For this review, take the finished solid that the model builds, in its own axes (mm). Round coordinates to 2 decimals unless told otherwise and drop trailing zeros. Order: outer loops, then holes, each group sorted by start corner. A loop starts at its lowest first (then second) coordinate and runs counter-clockwise, first axis right, second up. Notation, with made-up numbers: (61, -10.5) - (112, -10.5) arc R14 cw to (112, 5.5) - close; hole circle Ø7 at (-23, 53.5). An arc over 180 degrees is marked (long way). One line per question, with ' | ' between items.
```python
from build123d import *

# Parameters (mm, degrees)
SKETCH1_R           = 6
BOSS_EXTRUDE1_DEPTH = 6


with BuildPart() as part:
    # Sketch1 → Boss-Extrude1 (new body)
    with BuildSketch(Plane(origin=(0, 0, 0), x_dir=(1, 0, 0), z_dir=(0, 1, 0))):
        with BuildLine():
            Line((8.845195956, 114.659332409), (0, 0))
            Line((0, 0), (49.851883656, -3.845737372))
            Line((49.851883656, -3.845737372), (49.851883656, 10.382317327))
            Line((49.851883656, 10.382317327), (18.624081043, 115.696191659))
            ThreePointArc((18.624081043, 115.696191659), (13.303187452, 119.246887337), (8.845195956, 114.659332409))
        make_face()
        with Locations((16.515553245, 88.289115087)):
            Circle(SKETCH1_R, mode=Mode.SUBTRACT)
    extrude(amount=BOSS_EXTRUDE1_DEPTH)


solid = part.part
```
(1) Insertion check: pin 1 (3 mm diameter, centred on y = 4.5, z = -40.5, fed in from +X). The pin has a flat end and moves straight along its axis. Give the tip position at first contact, or say it passes through.
Output values:
pin 1: x = 41.37
(2) For probe 1 along X at (y, z) = (0.9, -89); probe 2 along X at (y, z) = (0.8, -85.5); probe 3 along Z at (x, y) = (12.5, 0.95), list the stretches that pass through material, from the lowest coordinate up. Write a range as [from, to].
Output values:
probe 1: [6.87, 10.56], [22.47, 26.54] | probe 2: [6.6, 11.2], [21.83, 27.58] | probe 3: [-119.09, -92.75], [-83.83, 0.96]
(3) We need section A-A on x = 21. State the section outline as (y, z) points.
Output values:
outline: (0, -107.68) - (6, -107.68) - (6, -92.28) - (0, -92.28) - close; (0, -84.3) - (6, -84.3) - (6, 1.62) - (0, 1.62) - close
(4) We need section C-C on z = -15. State the section outline as (x, y) points, plus the area to 3 significant figures.
Output values:
outline: (1.16, 0) - (48.48, 0) - (48.48, 6) - (1.16, 6) - close | area: 284 mm^2
(5) Mouldability with a two-part tool opening along X and no side actions: class faces 1 (the flat face through (19, 6, -45)), 2 (the flat face through (34.457, 2.958, -62.302)), 3 (the cylindrical face through (13.4, 2.958, -119.256)), 4 (the cylindrical face through (15.734, 2.958, -94.238)) as released by +X, released by -X, zero draft, split by the parting line, or undercut.
Output values:
face 1: zero draft | face 2: released by +X | face 3: split by the parting line | face 4: undercut
(6) We need section D-D on x = 4. State the section outline as (y, z) points, plus the area to 3 significant figures.
Output values:
outline: (0, -51.85) - (6, -51.85) - (6, 0.31) - (0, 0.31) - close | area: 313 mm^2
(7) We need section B-B on y = 4.25. State the section outline as (x, z) points, plus the area to 3 significant figures.
Output values:
outline: (0, 0) - (8.85, -114.66) arc R5 ccw to (18.62, -115.7) - (49.85, -10.38) - (49.85, 3.85) - close; hole circle Ø12 at (16.52, -88.29) | area: 3,610 mm^2
